Input: part model. Units: mm. Frame: model coordinates. A direction names the side the tool comes from. Coordinates: 2 decimals unless noted, no trailing zeros. Loops run counter-clockwise (first coordinate to the right, second up) from the corner with the lowest first, then second, coordinate; pieces in that order, holes last. Notation, with made-up numbers: (43, 29.5) - (72, 29.5) arc R16 ccw to (72, 52.5) - close; hole circle Ø7 at (-3.75, 12.5). An arc over 180 degrees is marked (long way). Use one line per item in the form item = value.
from build123d import *

# Parameters (mm, degrees)
F0_R      = 30
F1_DEPTH  = 14
F2_R      = 12
F3_DEPTH  = 20
F4_R      = 6
F5_DEPTH  = 25
F6_R      = 5
F7_DEPTH  = 34.001
F8_R      = 5
F9_DEPTH  = 34.001
F10_R     = 5
F11_DEPTH = 34.001
F12_R     = 5
F13_DEPTH = 34.001


with BuildPart() as f1:
    # F0 (on Top) → F1 (new body)
    with BuildSketch(Plane.XY):
        Circle(F0_R)
    extrude(amount=F1_DEPTH)

    # F2 (on face) → F3 (join)
    with BuildSketch(Plane.XY.offset(14)):
        Circle(F2_R)
    extrude(amount=F3_DEPTH)

    # F4 (on face) → F5 (cut)
    with BuildSketch(Plane.XY.offset(34)):
        Circle(F4_R)
    extrude(amount=-F5_DEPTH, mode=Mode.SUBTRACT)

    # F6 (on face) → F7 (cut, through all)
    with BuildSketch(Plane(origin=(0, 0, 0), x_dir=(1, 0, 0), z_dir=(0, 0, -1))):
        with Locations((0, -22.5)):
            Circle(F6_R)
    extrude(amount=-F7_DEPTH, mode=Mode.SUBTRACT)

    # F8 (on face) → F9 (cut, through all)
    with BuildSketch(Plane(origin=(0, 0, 0), x_dir=(1, 0, 0), z_dir=(0, 0, -1))):
        with Locations((0, 22.5)):
            Circle(F8_R)
    extrude(amount=-F9_DEPTH, mode=Mode.SUBTRACT)

    # F10 (on face) → F11 (cut, through all)
    with BuildSketch(Plane(origin=(0, 0, 0), x_dir=(1, 0, 0), z_dir=(0, 0, -1))):
        with Locations((-22.5, 0)):
            Circle(F10_R)
    extrude(amount=-F11_DEPTH, mode=Mode.SUBTRACT)

    # F12 (on face) → F13 (cut, through all)
    with BuildSketch(Plane(origin=(0, 0, 0), x_dir=(1, 0, 0), z_dir=(0, 0, -1))):
        with Locations((22.5, 0)):
            Circle(F12_R)
    extrude(amount=-F13_DEPTH, mode=Mode.SUBTRACT)


solid = f1.part
Q1. Cut plane B-B, the plane x = -22.5. Return loops of the section in (y, z), then the cut area to 3 significant figures.
Check values:
outline = (-19.84, 0) - (-5, 0) - (-5, 14) - (-19.84, 14) - close; (5, 0) - (19.84, 0) - (19.84, 14) - (5, 14) - close
area = 416 mm²
Q2. Pull-direction query (X, two-part tool) for faces 3 (the flat face through (-6, -2, 34)), 4 (the cylindrical face through (-27.495, -0.22, 6.902)), 5 (the cylindrical face through (-29.97, 1.32, 6.9)); classes: pulls with the +X half, pulls with the -X half, needs draft (parallel to the pull), parting line crosses it, or undercut.
Check values:
face_3 = needs draft
face_4 = undercut
face_5 = parting line crosses it
Q3. Ray query, line 1 along Y through (x, z) = (0, 4); line 2 along Y through (x, z) = (0, 26); line 3 along Z through (x, y) = (-15, -18.5). Return the intervals inside material, ascending. Write a range as [from, to].
Check values:
line_1 = [-30, -27.5], [-17.5, 17.5], [27.5, 30]
line_2 = [-12, -6], [6, 12]
line_3 = [0, 14]
Q4. Set-up query: faces 1 (the cylindrical face through (-6, 0, 22)), 2 (the cylindrical face through (17.505, -0.22, 6.902)). Return all of +Z, -Z, +X, -X, +Y, -Y with unobstructed straight access to the full face (end or side cutting, diameter ignored); none if empty.
Check values:
face_1 = +Z
face_2 = +Z, -Z
Q5. Cut plane A-A, the plane z = 13. Return loops of the section in (x, y).
Check values:
outline = circle Ø60 at (0, 0); hole circle Ø10 at (-22.5, 0); hole circle Ø12 at (0, 0); hole circle Ø10 at (0, -22.5); hole circle Ø10 at (0, 22.5); hole circle Ø10 at (22.5, 0)
Q6. First-contact query: P1, Ø6, axis at x = 9, z = 11.5, coming from the +Y side; P2, Ø12, axis at x = 11, z = 12.5, coming from the +Y side; P3, Ø8, axis at y = 7.5, z = 24.5, coming from the +X side. Flat tips, straight axial feed; report the tip coordinate or a pass-through.
Check values:
P1 = 29.39
P2 = 29.58
P3 = 11.48
Q7. Cut plane D-D, the plane z = 7. Return loops of the section in (x, y).
Check values:
outline = circle Ø60 at (0, 0); hole circle Ø10 at (-22.5, 0); hole circle Ø10 at (0, -22.5); hole circle Ø10 at (0, 22.5); hole circle Ø10 at (22.5, 0)
